Check sheet for the modelled part. Datum: model origin and axes. Units: mm. Face numbers are marked on the shaded views. A direction names the side the tool comes from. Round coordinates to 2 decimals unless told otherwise and drop trailing zeros. Loops run counter-clockwise (first coordinate to the right, second up) from the corner with the lowest first, then second, coordinate; pieces in that order, holes last. Notation, with made-up numbers: (0, -2.75) -> (26, -2.75) arc R29 cw to (26, 26.25) -> close; hole circle Ø9 at (82, 89). An arc over 180 degrees is marked (long way). One line per item, written item: value. Start each with the question number.
1. Cross-section at D-D on x = -9. Record the cut outline in (y, z).
2. Go/stop test with flat-tipped pins: pin 1 (3 mm diameter, centred on x = -11.5, z = 4, fed in from +Y); pin 2 (4.5 mm diameter, centred on y = 47, z = 4.5, fed in from -X); pin 3 (5 mm diameter, centred on x = -33.5, z = 8.5, fed in from -Y); pin 4 (2 mm diameter, centred on x = -38, y = 72, fed in from -Z). Record where each tip stops, or that it passes through.
3. Cross-section at A-A on z = 9. Count the separate pieces of the cut face and the enclosed holes in it, then the cut area to 3 significant figures.
4. Cross-section at B-B on x = 0. Record the cut outline in (y, z).
5. Cross-section at C-C on y = 0. Record the cut outline in (x, z).
6. Material ranges on L1, parallel to Y at x = 0, z = 1.25; L2, parallel to Y at x = -22, z = 1.25; L3, parallel to X at y = 72, z = 1.25, recorded low to high.
7. Release check for a two-part mould opening along Y. For the marked faces 4, 5, 6 and 7 record: +Y half, -Y half, draft (parallel to the pull), parting line (faces both ways), or undercut.
8. Set-up check for the marked faces 1, 2 and 3: record each of +Z, -Z, +X, -X, +Y, -Y from which the full face is reachable in a straight line by a thin tool's end or side.
from build123d import *

# Parameters (mm, degrees)
ESBO_O1_R                = 4
ESBO_O1_W                = 11
ESBO_O1_H                = 4
RESSALTO_EXTRUS_O1_DEPTH = 13
RESSALTO_EXTRUS_O3_START = -36
RESSALTO_EXTRUS_O3_DEPTH = 10
CORTE_EXTRUS_O2_START    = -10
ESBO_O7_R                = 8
CORTE_EXTRUS_O2_DEPTH    = 2.3
CORTE_EXTRUS_O3_START    = -2.3
ESBO_O7_2_R              = 8
CORTE_EXTRUS_O3_DEPTH    = 2.3
ESBO_O8_W                = 5.6
ESBO_O8_H                = 2.5
CORTE_EXTRUS_O4_DEPTH    = 10
ESBO_O9_R                = 1.75
CORTE_EXTRUS_O5_DEPTH    = 90.578178146


with BuildPart() as part:
    # Esbo_o1 → Ressalto-extrus_o1 (new body)
    with BuildSketch(Plane.XY):
        with BuildLine():
            Line((4, 63.65571123), (4, 6.34428877))
            ThreePointArc((4, 6.34428877), (0, -7.5), (-4, 6.34428877))
            Line((-4, 6.34428877), (-4, 41))
            Line((-4, 41), (-19, 41))
            Line((-19, 41), (-19, 53))
            Line((-19, 53), (-19, 77))
            Line((-19, 77), (-2.692582404, 77))
            ThreePointArc((-2.692582404, 77), (6.704091727, 73.362313803), (4, 63.65571123))
        make_face()
        with Locations(Location((0, 70, 0), (0, 0, 180))):
            Circle(ESBO_O1_R, mode=Mode.SUBTRACT)
        with Locations(Location((0, 0, 0), (0, 0, 180))):
            Circle(ESBO_O1_R, mode=Mode.SUBTRACT)
        with Locations((-9.5, 47)):
            Rectangle(ESBO_O1_W, ESBO_O1_H, mode=Mode.SUBTRACT)
    extrude(amount=RESSALTO_EXTRUS_O1_DEPTH)

    # Esbo_o5 → Ressalto-extrus_o3 (add)
    with BuildSketch(Plane.XZ.offset(-41).offset(RESSALTO_EXTRUS_O3_START)):
        with BuildLine():
            Line((-21, 13), (-19, 13))
            Line((-19, 13), (-19, 0))
            Line((-19, 0), (-43, 0))
            Line((-43, 0), (-43, 13))
            Line((-43, 13), (-35.5, 13))
            ThreePointArc((-35.5, 13), (-30, 7.5), (-24.5, 13))
            Line((-24.5, 13), (-21, 13))
        make_face()
    extrude(amount=RESSALTO_EXTRUS_O3_DEPTH)

    # Esbo_o7 → Corte-extrus_o2 (cut)
    with BuildSketch(Plane(origin=(0, 77, 0), x_dir=(1, 0, 0), z_dir=(0, 1, 0)).offset(CORTE_EXTRUS_O2_START)):
        with Locations((-30, -13)):
            Circle(ESBO_O7_R)
    extrude(amount=CORTE_EXTRUS_O2_DEPTH, mode=Mode.SUBTRACT)

    # Esbo_o7_2 → Corte-extrus_o3 (cut)
    with BuildSketch(Plane(origin=(0, 77, 0), x_dir=(1, 0, 0), z_dir=(0, 1, 0)).offset(CORTE_EXTRUS_O3_START)):
        with Locations((-30, -13)):
            Circle(ESBO_O7_2_R)
    extrude(amount=CORTE_EXTRUS_O3_DEPTH, mode=Mode.SUBTRACT)

    # Esbo_o8 → Corte-extrus_o4 (cut)
    with BuildSketch(Plane(origin=(0, 77, 0), x_dir=(1, 0, 0), z_dir=(0, 1, 0))):
        with Locations((-38, -4)):
            Rectangle(ESBO_O8_W, ESBO_O8_H)
        with Locations((-22, -4)):
            Rectangle(ESBO_O8_W, ESBO_O8_H)
    extrude(amount=-CORTE_EXTRUS_O4_DEPTH, mode=Mode.SUBTRACT)

    # Esbo_o9 → Corte-extrus_o5 (cut, through all)
    with BuildSketch(Plane.XY.offset(13)):
        with Locations((-38, 72)):
            Circle(ESBO_O9_R)
        with Locations((-22, 72)):
            Circle(ESBO_O9_R)
    extrude(amount=-CORTE_EXTRUS_O5_DEPTH, mode=Mode.SUBTRACT)


solid = part.part
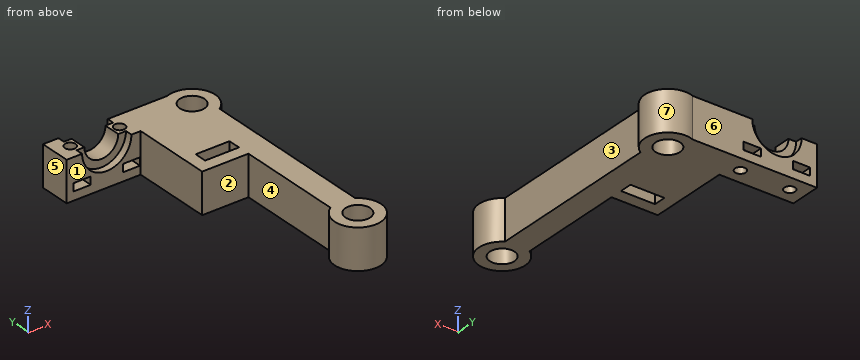
Taken from the geometry:
1. outline: (41, 0) -> (45, 0) -> (45, 13) -> (41, 13) -> close; (49, 0) -> (77, 0) -> (77, 13) -> (49, 13) -> close
2. pin 1: stops at y = 77
2. pin 2: stops at x = -19
2. pin 3: stops at y = 67
2. pin 4: passes through
3. separate pieces: 2
3. enclosed holes: 5
3. area: 1,280 mm2
4. outline: (-7.5, 0) -> (-4, 0) -> (-4, 13) -> (-7.5, 13) -> close; (4, 0) -> (66, 0) -> (66, 13) -> (4, 13) -> close; (74, 0) -> (77.5, 0) -> (77.5, 13) -> (74, 13) -> close
5. outline: (-7.5, 0) -> (-4, 0) -> (-4, 13) -> (-7.5, 13) -> close; (4, 0) -> (7.5, 0) -> (7.5, 13) -> (4, 13) -> close
6. L1: y = -7.5 to -4, 4 to 66, 74 to 77.5
6. L2: y = 67 to 70.25, 73.75 to 77
6. L3: x = -43 to -39.75, -36.25 to -23.75, -20.25 to -3.46, 3.46 to 7.23
7. face 4: undercut
7. face 5: draft
7. face 6: +Y half
7. face 7: undercut
8. face 1: +Z, -Z, -X, -Y
8. face 2: +Z, -Z, -X
8. face 3: +Z, -Z, +X
